For this review, take the finished solid that the model builds, in its own axes (mm). Face numbers are marked on the shaded views. Round coordinates to 2 decimals unless told otherwise and drop trailing zeros. Order: outer loops, then holes, each group sorted by start corner. A loop starts at its lowest first (then second) coordinate and runs counter-clockwise, first axis right, second up.
```python
from build123d import *

# Parameters (mm, degrees)
F2_SIZE = 1


with BuildPart() as f1:
    # F0 (on Front) → F1 (revolve)
    with BuildSketch(Plane.XZ):
        Polygon((10, 20), (2.6, 20), (2.6, 0), (15, 0), (15, 5), align=None)
    revolve(axis=Axis((0, 0, 10), (0, 0, -1)))

    # F2
    f2_edges = [f1.edges().sort_by_distance(p)[0] for p in [
        (-2.6, 0, 20),
        (-2.6, 0, 0),
        (-15, 0, 0),
    ]]
    chamfer(f2_edges, length=F2_SIZE)


solid = f1.part
```
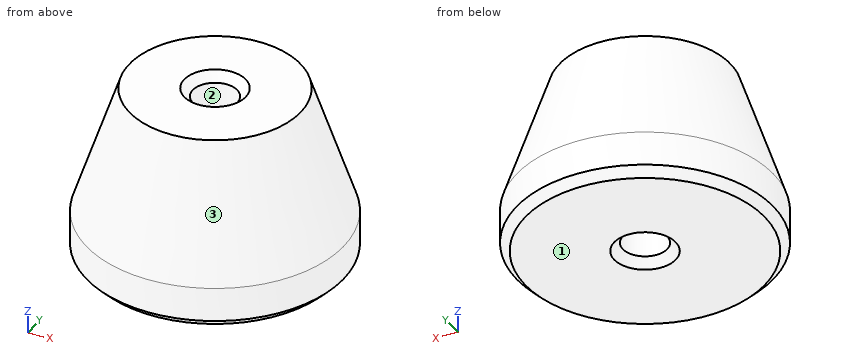
Q1. Take a section at C-C, the plane z = 15. State the section outline as (x, y) points, plus the area to 3 significant figures.
Q2. Mouldability with a two-part tool opening along X and no side actions: class the marked faces 1, 2 and 3 as +X half, -X half, draft (parallel to the pull), parting line (faces both ways), or undercut.
Q3. Take a section at A-A, the plane x = 0. State the section outline as (y, z) points, plus the area to 3 significant figures.
Q4. Take a section at D-D, the plane z = 18. State the section outline as (x, y) points, plus the area to 3 significant figures.
Q5. Wall thickness on line 1 (Y direction, x = 0, z = 12.25); line 2 (Y direction, x = 0, z = 11.5); line 3 (X direction, y = 0, z = 9.25): over which ranges is each line inside the solid? List them lowest first.
Q6. Clearance check with flat-ended pins moving along their axes: pin 1 (1.5 mm diameter, centred on y = -11, z = 13, fed in from +X); pin 2 (3 mm diameter, centred on x = 0, y = 0, fed in from -Z); pin 3 (12 mm diameter, centred on y = 8, z = 5, fed in from +X); pin 4 (5 mm diameter, centred on x = -5, z = 10.5, fed in from +Y). State where each tip first meets the part, or that it passes through.
Working result:
1. outline: circle Ø23.33 at (0, 0); hole circle Ø5.2 at (0, 0)
1. area: 406 mm2
2. face 1: draft
2. face 2: undercut
2. face 3: parting line
3. outline: (-15, 1) - (-14, 0) - (-3.6, 0) - (-2.6, 1) - (-2.6, 19) - (-3.6, 20) - (-10, 20) - (-15, 5) - close; (2.6, 1) - (3.6, 0) - (14, 0) - (15, 1) - (15, 5) - (10, 20) - (3.6, 20) - (2.6, 19) - close
3. area: 418 mm2
4. outline: circle Ø21.33 at (0, 0); hole circle Ø5.2 at (0, 0)
4. area: 336 mm2
5. line 1: y = -12.58 to -2.6, 2.6 to 12.58
5. line 2: y = -12.83 to -2.6, 2.6 to 12.83
5. line 3: x = -13.58 to -2.6, 2.6 to 13.58
6. pin 1: stops at x = 6.95
6. pin 2: passes through
6. pin 3: stops at x = 14.87
6. pin 4: stops at y = 13.38
